Design review of the part built by this model. Coordinates are the model's own, in mm. A direction names the side the tool comes from. Round coordinates to 2 decimals unless told otherwise and drop trailing zeros. Write each loop counter-clockwise with the first axis right and the second up, starting at its lowest first coordinate (ties: lowest second). Pieces come first, ordered by that corner, then holes. Notation, with made-up numbers: (67, 2.25) -> (101, 2.25) arc R20 cw to (101, 19.25) -> close; hole circle Ø7 at (83, 74). An arc over 180 degrees is marked (long way). One line per question, with ' | ' between items. Start each with the question number.
1) Mouldability with a two-part tool opening along Y and no side actions: class faces 1 (the flat face through (-16, -53, -134)), 2 (the cylindrical face through (-38.616, -39.944, -140.528)), 3 (the flat face through (-38.99, -39.53, -143.46)), 4 (the cylindrical face through (57, 0, -142)) as +Y half, -Y half, draft (parallel to the pull), parting line (faces both ways), or undercut.
2) For faces 5 (the flat face through (54, 12, -134)), 6 (the flat face through (-14.74, 53.53, -143.46)), 7 (the flat face through (-17.684, -52.629, -136.282)), 8 (the cylindrical face through (11.706, 52.716, -136.126)), list the 3-axis set-ups (+Z, -Z, +X, -X, +Y, -Y) from which the entire face can be reached by the end or side of a thin tool; tool diameter is ignored.
3) Insertion check: pin 1 Ø0.9 at (x, z) = (53, -144) entering from -Y; pin 2 Ø3.5 at (x, y) = (55, 13) entering from +Z; pin 3 Ø1.6 at (x, z) = (53.5, -139.5) entering from +Y. Each pin has a flat end and moves straight along its axis. Give the tip position at first contact, or say it passes through.
4) Consider section D-D (z = -132.5). Give the boundary of the cut face in (x, y).
5) For probe 1 along Y at (x, z) = (0, -133); probe 2 along Z at (x, y) = (-37.5, -41), list the stretches that pass through material, from the lowest coordinate up.
6) Consider section C-C (y = 16). Give the boundary of the cut face in (x, z), then the cut area to 3 significant figures.
7) Consider section A-A (y = 0). Give the boundary of the cut face in (x, z), then the cut area to 3 significant figures.
8) Consider section B-B (x = -8.5). Give the boundary of the cut face in (y, z).
```python
from build123d import *

# Parameters (mm, degrees)
EXTRUDE_1_DEPTH                  = 10
FILLET_1_R                       = 2
PATTERN_CIRCULAR_2_COUNT         = 3
FILLET_1_OF_PATTERN_CIRCULAR_2_R = 2
CUT_EXTRUDE_START                = -15
SKETCH_3_R                       = 51
CUT_EXTRUDE_1_DEPTH              = 15
SKETCH_4_R                       = 62.618720145
SKETCH_4_R_2                     = 57
CUT_EXTRUDE_2_DEPTH              = 15
CHAMFER_1_SIZE                   = 2
FILLET_2_R                       = 5
SKETCH_5_R                       = 42.5
EXTRUDE_2_DEPTH                  = 3
SKETCH_7_R                       = 39.5
CUT_EXTRUDE_3_DEPTH              = 3
EXTRUDE_START                    = 3
SKETCH_8_W                       = 3
SKETCH_8_H                       = 3
EXTRUDE_4_DEPTH                  = 3
SKETCH_11_R                      = 73.482680971
CUT_EXTRUDE_4_DEPTH              = 130


with BuildPart() as part:
    # Эскиз1 → Повернуть1 (revolve)
    with BuildSketch(Plane(origin=(0, 0, 0), x_dir=(1, 0, 0), z_dir=(0, 1, 0))):
        Polygon((0, 0), (-54, 0), (-54, 145), (-51, 145), (-51, 3), (0, 3), align=None)
    revolve(axis=Axis((0, 0, -3), (0, 0, 1)))

    # Эскиз2 → Бобышка-Вытянуть1 (add)
    with BuildSketch(Plane(origin=(57, 0, 0), x_dir=(0, 0, -1), z_dir=(1, 0, 0))):
        Polygon((145, 14), (145, -14), (140, -14), (138.5, 11), (134, 11), (134, 14), align=None)
    extrude_1 = extrude(amount=-EXTRUDE_1_DEPTH)

    # Скругление1
    fillet_1_edges = [part.edges().sort_by_distance(p)[0] for p in [
        (54.576809621, -14, -140),
    ]]
    fillet(fillet_1_edges, radius=FILLET_1_R)

    # Круговой массив2: Бобышка-Вытянуть1 ×3 about axis
    pattern_circular_2_axis = Axis((0, 0, 0), (0, 0, 1))
    for i in range(1, PATTERN_CIRCULAR_2_COUNT):
        add(extrude_1.rotate(pattern_circular_2_axis, i * 360 / PATTERN_CIRCULAR_2_COUNT))

    # Скругление1 of Круговой массив2
    fillet_1_of_pattern_circular_2_edges = [part.edges().sort_by_distance(p)[0] for p in [
        (-15.164049157, 54.264903589, -140),
        (-39.412760463, -40.264903589, -140),
    ]]
    fillet(fillet_1_of_pattern_circular_2_edges, radius=FILLET_1_OF_PATTERN_CIRCULAR_2_R)

    # Эскиз3 → Вырез-Вытянуть1 (cut)
    with BuildSketch(Plane(origin=(0, 0, -145), x_dir=(-1, 0, 0), z_dir=(0, 0, -1)).offset(CUT_EXTRUDE_START)):
        Circle(SKETCH_3_R)
    extrude(amount=CUT_EXTRUDE_1_DEPTH, mode=Mode.SUBTRACT)

    # Эскиз4 → Вырез-Вытянуть2 (cut)
    with BuildSketch(Plane(origin=(0, 0, -145), x_dir=(-1, 0, 0), z_dir=(0, 0, -1))):
        Circle(SKETCH_4_R)
        Circle(SKETCH_4_R_2, mode=Mode.SUBTRACT)
    extrude(amount=-CUT_EXTRUDE_2_DEPTH, mode=Mode.SUBTRACT)

    # Фаска1
    chamfer_1_edges = [part.edges().sort_by_distance(p)[0] for p in [
        (54, 0, 0),
    ]]
    chamfer(chamfer_1_edges, length=CHAMFER_1_SIZE)

    # Скругление2
    fillet_2_edges = [part.edges().sort_by_distance(p)[0] for p in [
        (51, 0, -3),
    ]]
    fillet(fillet_2_edges, radius=FILLET_2_R)

    # Эскиз5 → Бобышка-Вытянуть2 (add)
    with BuildSketch(Plane.XY):
        Circle(SKETCH_5_R)
    extrude(amount=EXTRUDE_2_DEPTH)

    # Эскиз7 → Вырез-Вытянуть3 (cut)
    with BuildSketch(Plane.XY.offset(3)):
        Circle(SKETCH_7_R)
    extrude(amount=-CUT_EXTRUDE_3_DEPTH, mode=Mode.SUBTRACT)

    # Эскиз8 → Бобышка-Вытянуть4 (add)
    with BuildSketch(Plane.XY.offset(EXTRUDE_START)):
        with BuildLine():
            Line((-1.5, -7.858116823), (-1.5, -39.471508712))
            ThreePointArc((-1.5, -39.471508712), (0, -39.5), (1.5, -39.471508712))
            Line((1.5, -39.471508712), (1.5, -7.858116823))
            ThreePointArc((1.5, -7.858116823), (0, -8), (-1.5, -7.858116823))
        make_face()
        with BuildLine():
            ThreePointArc((1.5, 39.471508712), (0, 39.5), (-1.5, 39.471508712))
            Line((-1.5, 39.471508712), (-1.5, 7.858116823))
            ThreePointArc((-1.5, 7.858116823), (0, 8), (1.5, 7.858116823))
            Line((1.5, 7.858116823), (1.5, 39.471508712))
        make_face()
        with BuildLine():
            Line((-1.5, 7.858116823), (-1.5, 1.5))
            Line((-1.5, 1.5), (1.5, 1.5))
            Line((1.5, 1.5), (1.5, 7.858116823))
            ThreePointArc((1.5, 7.858116823), (0, 8), (-1.5, 7.858116823))
        make_face()
        with BuildLine():
            Line((1.5, 7.858116823), (1.5, 1.5))
            Line((1.5, 1.5), (7.858116823, 1.5))
            ThreePointArc((7.858116823, 1.5), (5.656854249, 5.656854249), (1.5, 7.858116823))
        make_face()
        with BuildLine():
            Line((1.5, 1.5), (1.5, -1.5))
            Line((1.5, -1.5), (7.858116823, -1.5))
            ThreePointArc((7.858116823, -1.5), (7.964450219, -0.753347668), (8, 0))
            ThreePointArc((8, 0), (7.964450219, 0.753347668), (7.858116823, 1.5))
            Line((7.858116823, 1.5), (1.5, 1.5))
        make_face()
        with BuildLine():
            ThreePointArc((-39.471508712, 1.5), (-39.5, 0), (-39.471508712, -1.5))
            Line((-39.471508712, -1.5), (-7.858116823, -1.5))
            ThreePointArc((-7.858116823, -1.5), (-8, 0), (-7.858116823, 1.5))
            Line((-7.858116823, 1.5), (-39.471508712, 1.5))
        make_face()
        with BuildLine():
            Line((7.858116823, -1.5), (39.471508712, -1.5))
            ThreePointArc((39.471508712, -1.5), (39.492876536, -0.75013528), (39.5, 0))
            ThreePointArc((39.5, 0), (39.492876536, 0.75013528), (39.471508712, 1.5))
            Line((39.471508712, 1.5), (7.858116823, 1.5))
            ThreePointArc((7.858116823, 1.5), (7.964450219, 0.753347668), (8, 0))
            ThreePointArc((8, 0), (7.964450219, -0.753347668), (7.858116823, -1.5))
        make_face()
        with BuildLine():
            Line((1.5, -1.5), (1.5, -7.858116823))
            ThreePointArc((1.5, -7.858116823), (5.656854249, -5.656854249), (7.858116823, -1.5))
            Line((7.858116823, -1.5), (1.5, -1.5))
        make_face()
        with BuildLine():
            Line((-1.5, -1.5), (-1.5, -7.858116823))
            ThreePointArc((-1.5, -7.858116823), (0, -8), (1.5, -7.858116823))
            Line((1.5, -7.858116823), (1.5, -1.5))
            Line((1.5, -1.5), (-1.5, -1.5))
        make_face()
        Rectangle(SKETCH_8_W, SKETCH_8_H)
        with BuildLine():
            Line((-7.858116823, 1.5), (-1.5, 1.5))
            Line((-1.5, 1.5), (-1.5, 7.858116823))
            ThreePointArc((-1.5, 7.858116823), (-5.656854249, 5.656854249), (-7.858116823, 1.5))
        make_face()
        with BuildLine():
            Line((-7.858116823, -1.5), (-1.5, -1.5))
            Line((-1.5, -1.5), (-1.5, 1.5))
            Line((-1.5, 1.5), (-7.858116823, 1.5))
            ThreePointArc((-7.858116823, 1.5), (-8, 0), (-7.858116823, -1.5))
        make_face()
        with BuildLine():
            ThreePointArc((-7.858116823, -1.5), (-5.656854249, -5.656854249), (-1.5, -7.858116823))
            Line((-1.5, -7.858116823), (-1.5, -1.5))
            Line((-1.5, -1.5), (-7.858116823, -1.5))
        make_face()
    extrude(amount=-EXTRUDE_4_DEPTH)

    # Эскиз11 → Вырез-Вытянуть4 (cut)
    with BuildSketch(Plane.XY.offset(3)):
        Circle(SKETCH_11_R)
    extrude(amount=-CUT_EXTRUDE_4_DEPTH, mode=Mode.SUBTRACT)


solid = part.part
```
From the geometry:
1) face 1: draft | face 2: undercut | face 3: undercut | face 4: parting line
2) face 5: +Z, +X, +Y | face 6: +Z, -Z, +Y | face 7: +Z, -X | face 8: +Z
3) pin 1: stops at y = -14 | pin 2: stops at z = -134 | pin 3: stops at y = 14
4) outline: circle Ø108 at (0, 0); hole circle Ø102 at (0, 0)
5) probe 1: y = -54 to -51, 51 to 54 | probe 2: z = -145 to -139.88
6) outline: (-51.58, -145) -> (-48.43, -145) -> (-48.43, -127) -> (-51.58, -127) -> close; (48.43, -145) -> (51.58, -145) -> (51.58, -127) -> (48.43, -127) -> close | area: 113 mm2
7) outline: (-54, -145) -> (-51, -145) -> (-51, -127) -> (-54, -127) -> close; (51, -145) -> (57, -145) -> (57, -139.16) -> (54, -139.16) -> (54, -127) -> (51, -127) -> close | area: 126 mm2
8) outline: (-53.33, -145) -> (-50.29, -145) -> (-50.29, -127) -> (-53.33, -127) -> close; (50.29, -145) -> (53.33, -145) -> (53.33, -127) -> (50.29, -127) -> close
